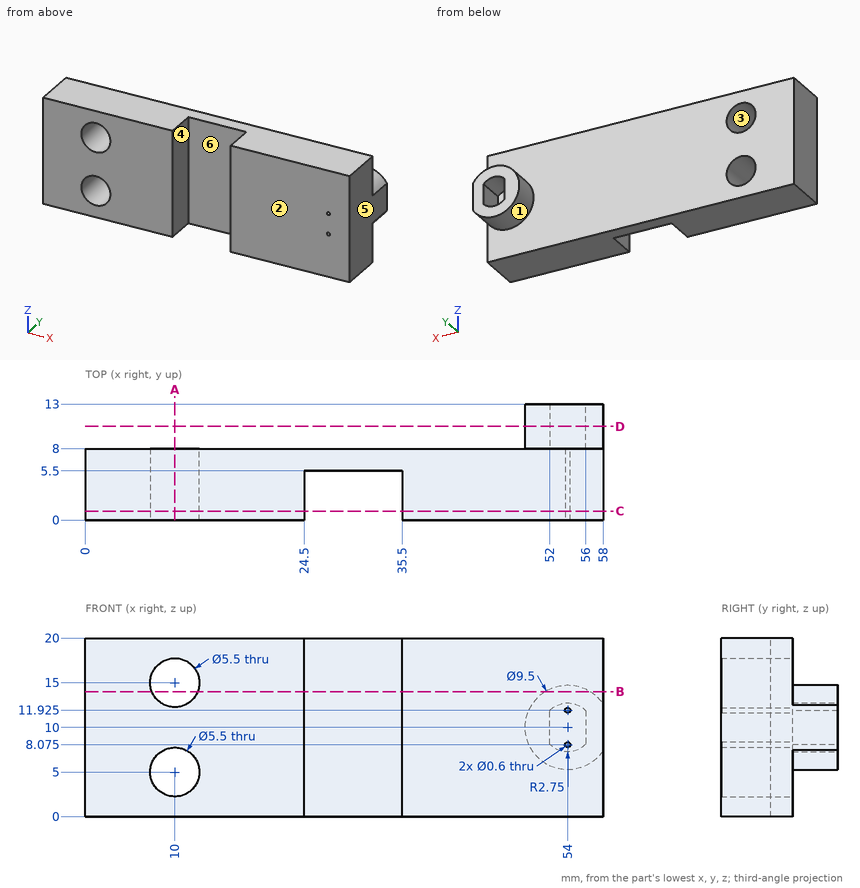
Input: dimensioned drawing with shaded views. Units: mm. Origin: part minimum x, y, z. A direction names the side the tool comes from. Give positions to 0.01 mm unless a question says otherwise; leave off trailing zeros. Write each loop counter-clockwise with the first axis right and the second up, starting at its lowest first coordinate (ties: lowest second). Pieces come first, ordered by that corner, then holes.
Q1. First-contact query: P1, Ø3, axis at y = 11, z = 10, coming from the -X side; P2, Ø7, axis at x = 10, z = 15, coming from the +Y side; P3, Ø3.5, axis at x = 10, z = 5, coming from the +Y side. Flat tips, straight axial feed; report the tip coordinate or a pass-through.
Q2. Section B-B, the plane z = 14. Output: boundary loops of the cut face in (x, y), plus the area to 3 significant figures.
Q3. Section D-D, the plane y = 10.5. Output: boundary loops of the cut face in (x, z), plus the area to 3 significant figures.
Q4. Material intervals for probe 1 along Z at (x, y) = (10, 2.5); probe 2 along Z at (x, y) = (54, 6.5) (3 decimals); probe 3 along X at (y, z) = (4.5, 18), sorted ascending.
Q5. Section C-C, the plane y = 1. Output: boundary loops of the cut face in (x, z) (3 decimals).
Q6. Set-up query: the marked faces 5 and 6. Return all of +Z, -Z, +X, -X, +Y, -Y with unobstructed straight access to the full face (end or side cutting, diameter ignored); none if empty.
Q7. Pull-direction query (X, two-part tool) for the marked faces 1, 2, 3 and 4; classes: pulls with the +X half, pulls with the -X half, needs draft (parallel to the pull), parting line crosses it, or undercut.
Q8. Section A-A, the plane x = 10. Output: boundary loops of the cut face in (y, z).
Filled in:
1. P1: stops at x = 49.25
1. P2: stops at y = 8
1. P3: passes through
2. outline: (0, 0) - (7.44, 0) - (7.44, 8) - (0, 8) - close; (12.56, 0) - (24.5, 0) - (24.5, 5.5) - (35.5, 5.5) - (35.5, 0) - (58, 0) - (58, 8) - (56.56, 8) - (56.56, 13) - (51.44, 13) - (51.44, 8) - (12.56, 8) - close
2. area: 388 mm2
3. outline: (58, 7.44) - (58, 12.56) arc R4.75 ccw (long way) to start; hole (52, 8.11) arc R2.75 ccw to (56, 8.11) - (56, 11.89) arc R2.75 ccw to (52, 11.89) - close
3. area: 48.4 mm2
4. probe 1: z = 0 to 2.25, 7.75 to 12.25, 17.75 to 20
4. probe 2: z = 0 to 7.775, 8.375 to 11.625, 12.225 to 20
4. probe 3: x = 0 to 24.5, 35.5 to 58
5. outline: (0, 0) - (24.5, 0) - (24.5, 20) - (0, 20) - close; (35.5, 0) - (58, 0) - (58, 20) - (35.5, 20) - close; hole circle Ø5.5 at (10, 5); hole circle Ø5.5 at (10, 15); hole circle Ø0.6 at (54, 8.075); hole circle Ø0.6 at (54, 11.925)
6. face 5: +Z, -Z, +X, +Y, -Y
6. face 6: +Z, -Z, -Y
7. face 1: parting line crosses it
7. face 2: needs draft
7. face 3: undercut
7. face 4: undercut
8. outline: (0, 0) - (8, 0) - (8, 2.25) - (0, 2.25) - close; (0, 7.75) - (8, 7.75) - (8, 12.25) - (0, 12.25) - close; (0, 17.75) - (8, 17.75) - (8, 20) - (0, 20) - close
